Geometry check sheet. Reference: the model listing, model coordinates, mm. Face numbers are marked on the shaded views. Round coordinates to 2 decimals unless told otherwise and drop trailing zeros. Order: outer loops, then holes, each group sorted by start corner. A loop starts at its lowest first (then second) coordinate and runs counter-clockwise, first axis right, second up.
(1) Release check for a two-part mould opening along Z. For the marked faces 1, 2 and 3 record: +Z half, -Z half, draft (parallel to the pull), parting line (faces both ways), or undercut.
(2) Sectioned sample at B-B (z = 0). Record the boundary of the cut face in (x, y), plus the area to 3 significant figures.
(3) Go/stop test with flat-tipped pins: pin 1 (4 mm diameter, centred on x = -6, y = 5.5, fed in from +Z); pin 2 (10 mm diameter, centred on x = 11, y = 3, fed in from -Z); pin 3 (3 mm diameter, centred on x = -9, y = 10, fed in from -Z). Record where each tip stops, or that it passes through.
(4) Sectioned sample at C-C (y = 1.5). Record the boundary of the cut face in (x, z), plus the area to 3 significant figures.
(5) Material ranges on line 1 along Z through (x, y) = (0, 3.5); line 2 along Y through (x, z) = (-3, 12.5); line 3 along X through (y, z) = (-9, 3), recorded low to high.
(6) Sectioned sample at A-A (x = 0). Record the boundary of the cut face in (y, z).
Autodesk Fusion 360 part; units mm, degrees
sketch "Sketch1" plane through (0, 0, 0) normal (0, 1, 0) x (1, 0, 0)
  circle A0 centre (0, 0) radius 15.24
  dimension "d1" = 30.48
extrude "Extrude1" add sketch "Sketch1" along normal mid plane 38.1
fillet "Fillet1" radius 2.54 2 edges at (-14.2087, -19.05, -5.511) (-14.2087, 19.05, 5.511)
sketch "Sketch2" plane through (0, -19.05, 0) normal (0, -1, 0) x (1, 0, 0)
  circle A0 centre (0, 0) radius 12.7
  circle A1 centre (0, 0) radius 3.81
  dimension "d6" = 7.62
extrude "Extrude2" cut sketch "Sketch2" against normal through all contours A1
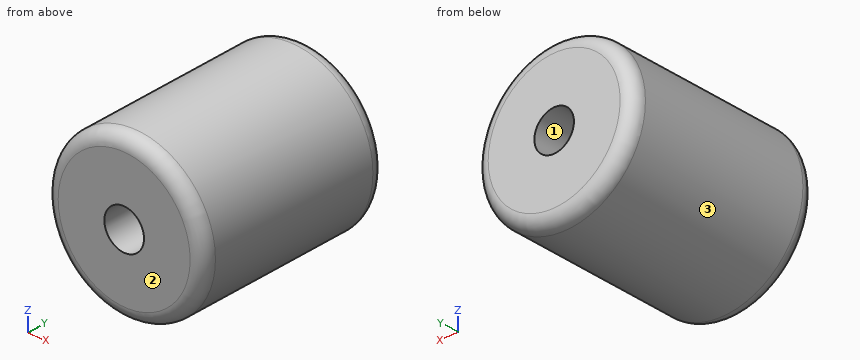
Answer below:
1. face 1: undercut
1. face 2: draft
1. face 3: parting line
2. outline: (-15.24, -16.51) arc R2.54 ccw to (-12.7, -19.05) - (-3.81, -19.05) - (-3.81, 19.05) - (-12.7, 19.05) arc R2.54 ccw to (-15.24, 16.51) - close; (3.81, -19.05) - (12.7, -19.05) arc R2.54 ccw to (15.24, -16.51) - (15.24, 16.51) arc R2.54 ccw to (12.7, 19.05) - (3.81, 19.05) - close
2. area: 865 mm2
3. pin 1: stops at z = 14.71
3. pin 2: stops at z = -14.01
3. pin 3: stops at z = -13.27
4. outline: circle Ø30.48 at (0, 0); hole circle Ø7.62 at (0, 0)
4. area: 684 mm2
5. line 1: z = -15.24 to -3.81, 3.81 to 15.24
5. line 2: y = -19.05 to 19.05
5. line 3: x = -14.94 to -2.35, 2.35 to 14.94
6. outline: (-19.05, -12.7) arc R2.54 ccw to (-16.51, -15.24) - (16.51, -15.24) arc R2.54 ccw to (19.05, -12.7) - (19.05, -3.81) - (-19.05, -3.81) - close; (-19.05, 3.81) - (19.05, 3.81) - (19.05, 12.7) arc R2.54 ccw to (16.51, 15.24) - (-16.51, 15.24) arc R2.54 ccw to (-19.05, 12.7) - close
